Verification items for the finished model (mm, model axes). A direction names the side the tool comes from. Coordinates: 2 decimals unless noted, no trailing zeros. Write each loop counter-clockwise with the first axis right and the second up, starting at its lowest first coordinate (ties: lowest second). Pieces come first, ordered by that corner, then holes. Notation, with made-up numbers: (19, 66.5) -> (57, 66.5) arc R15 ccw to (57, 81.5) -> close; hole circle Ø7 at (18, 79). An arc over 180 degrees is marked (long way). Use CSV: the item, a comma, the result in double quotes.
```python
from build123d import *

# Parameters (mm, degrees)
SKETCH_1_W          = 25
SKETCH_1_H          = 76
EXTRUDE_1_DEPTH     = 14
SKETCH_2_W          = 3
SKETCH_2_H          = 10
EXTRUDE_2_DEPTH     = 55
SKETCH_3_R          = 2.1
CUT_EXTRUDE_1_DEPTH = 69.009190555
CUT_EXTRUDE_3_DEPTH = 69.009190555
SKETCH_6_R          = 3
CUT_EXTRUDE_4_DEPTH = 5


with BuildPart() as part:
    # 草图1 → 凸台-拉伸1 (new body)
    with BuildSketch(Plane.XY):
        Rectangle(SKETCH_1_W, SKETCH_1_H)
    extrude(amount=EXTRUDE_1_DEPTH)

    # 草图2 → 凸台-拉伸2 (add)
    with BuildSketch(Plane.XY.offset(14)):
        Rectangle(SKETCH_2_W, SKETCH_2_H)
    extrude(amount=EXTRUDE_2_DEPTH)

    # 草图3 → 切除-拉伸1 (cut, through all)
    with BuildSketch(Plane.XY.offset(14)):
        with Locations((-7, -20)):
            Circle(SKETCH_3_R)
        with Locations((-7, -32)):
            Circle(SKETCH_3_R)
        with Locations(Location((7, -32, 0), (0, 0, 180))):
            Circle(SKETCH_3_R)
        with Locations(Location((7, -20, 0), (0, 0, 180))):
            Circle(SKETCH_3_R)
    extrude(amount=-CUT_EXTRUDE_1_DEPTH, mode=Mode.SUBTRACT)

    # 草图5 → 切除-拉伸3 (cut, through all)
    with BuildSketch(Plane.XY.offset(14)):
        with BuildLine():
            Line((-7, 13), (7, 13))
            Line((7, 13), (7, 27))
            ThreePointArc((7, 27), (1.5, 32.5), (7, 38))
            Line((7, 38), (-7, 38))
            ThreePointArc((-7, 38), (-1.5, 32.5), (-7, 27))
            Line((-7, 27), (-7, 13))
        make_face()
    extrude(amount=-CUT_EXTRUDE_3_DEPTH, mode=Mode.SUBTRACT)

    # 草图6 → 切除-拉伸4 (cut)
    with BuildSketch(Plane(origin=(0, 0, 0), x_dir=(-1, 0, 0), z_dir=(0, 0, -1))):
        with Locations((7, -20)):
            Circle(SKETCH_6_R)
        with Locations((-7, -20)):
            Circle(SKETCH_6_R)
        with Locations((-7, -32)):
            Circle(SKETCH_6_R)
        with Locations((7, -32)):
            Circle(SKETCH_6_R)
    extrude(amount=-CUT_EXTRUDE_4_DEPTH, mode=Mode.SUBTRACT)


solid = part.part
```
1) Set-up check for faces 1 (the flat face through (0, 5, 41)), 2 (the flat face through (0, -5, 41)), 3 (the flat face through (7, 20, 7)), 4 (the flat face through (5.7, -34, 5)): record each of +Z, -Z, +X, -X, +Y, -Y from which the full face is reachable in a straight line by a thin tool's end or side.
Return value:
face 1,"+Z, +X, -X, +Y"
face 2,"+Z, +X, -X, -Y"
face 3,"+Z, -Z"
face 4,"-Z"
2) Mould release check, pull along Y, two halves, no side actions. Record for faces 5 (the cylindrical face through (-7.273, -17.918, 9.563)), 6 (the flat face through (0, 1, 0)), 7 (the flat face through (-10, 38, 7)): released by +Y, released by -Y, zero draft, split by the parting line, or undercut.
Return value:
face 5,"undercut"
face 6,"zero draft"
face 7,"released by +Y"
3) Cross-section at D-D (z = 9). Record the boundary of the cut face in (x, y), plus the area to 3 significant figures.
Return value:
outline,"(-12.5, -38) -> (12.5, -38) -> (12.5, 38) -> (7, 38) arc R5.5 ccw to (7, 27) -> (7, 13) -> (-7, 13) -> (-7, 27) arc R5.5 ccw to (-7, 38) -> (-12.5, 38) -> close; hole circle Ø4.2 at (-7, -32); hole circle Ø4.2 at (-7, -20); hole circle Ø4.2 at (7, -32); hole circle Ø4.2 at (7, -20)"
area,"1,590 mm2"
4) Scan lines: L1, parallel to X at y = -19, z = 4; L2, parallel to Z at x = -10.5, y = 5; L3, parallel to Z at x = -8.5, y = -34. Record each from-to range of solid material in increasing order.
Return value:
L1,"-12.5 to -9.83, -4.17 to 4.17, 9.83 to 12.5"
L2,"0 to 14"
L3,"5 to 14"
5) Gauge pin test, flat ends, axial feed: pin 1 (5 mm diameter, centred on y = 1.5, z = 50.5, fed in from -X); pin 2 (1.8 mm diameter, centred on x = 5.5, y = -31.5, fed in from -Z); pin 3 (1 mm diameter, centred on x = 2.5, z = 8, fed in from +Y). Record the tip position at first contact, or that the pin passes through.
Return value:
pin 1,"x = -1.5"
pin 2,"z = 5"
pin 3,"y = 36.27"
6) Cross-section at C-C (y = 32.5). Record the boundary of the cut face in (x, z).
Return value:
outline,"(-12.5, 0) -> (-1.5, 0) -> (-1.5, 14) -> (-12.5, 14) -> close; (1.5, 0) -> (12.5, 0) -> (12.5, 14) -> (1.5, 14) -> close"
7) Cross-section at B-B (x = -2.5). Record the boundary of the cut face in (y, z).
Return value:
outline,"(-38, 0) -> (13, 0) -> (13, 14) -> (-38, 14) -> close; (29.34, 0) -> (35.66, 0) -> (35.66, 14) -> (29.34, 14) -> close"
8) Cross-section at A-A (y = -32). Record the boundary of the cut face in (x, z).
Return value:
outline,"(-12.5, 0) -> (-10, 0) -> (-10, 5) -> (-9.1, 5) -> (-9.1, 14) -> (-12.5, 14) -> close; (-4.9, 5) -> (-4, 5) -> (-4, 0) -> (4, 0) -> (4, 5) -> (4.9, 5) -> (4.9, 14) -> (-4.9, 14) -> close; (9.1, 5) -> (10, 5) -> (10, 0) -> (12.5, 0) -> (12.5, 14) -> (9.1, 14) -> close"
